Can you work these out from the model? Positions are in its coordinate system, mm. Face numbers are marked on the shaded views. A direction names the side the tool comes from. Round coordinates to 2 decimals unless told otherwise and drop trailing zeros. Loops run counter-clockwise (first coordinate to the right, second up) from the corner with the lowest first, then second, coordinate; pieces in that order, holes last. Notation, with made-up numbers: M 36.25,21.5 L 82.25,21.5 A26 ccw 82.25,56.5 Z; hole C 75,-37 d6. An arc over 180 degrees is marked long. Return JSON: item names as keys, results as strings.
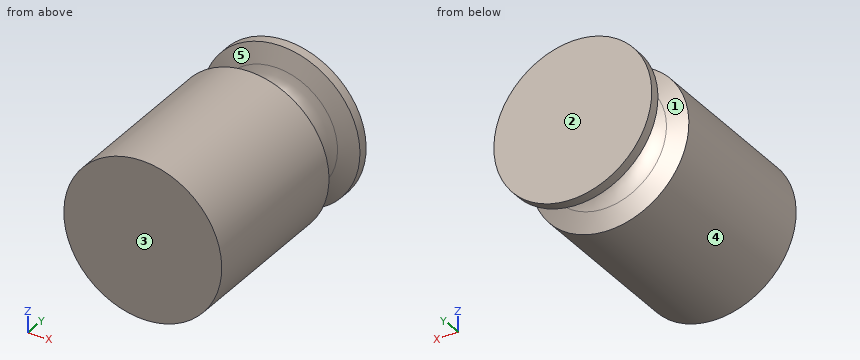
```python
from build123d import *

# Parameters (mm, degrees)
SKETCH1_R           = 25
BOSS_EXTRUDE1_DEPTH = 70


with BuildPart() as part:
    # Sketch1 → Boss-Extrude1 (new body)
    with BuildSketch(Plane(origin=(0, 0, 0), x_dir=(1, 0, 0), z_dir=(0, 1, 0))):
        with Locations(Location((0, 0, 0), (0, 0, 270))):
            Circle(SKETCH1_R)
    extrude(amount=BOSS_EXTRUDE1_DEPTH)

    # Sketch2 → Cut-Revolve3 (revolve, cut)
    with BuildSketch(Plane.XY, mode=Mode.PRIVATE) as cut_revolve3_sk:
        with BuildLine():
            Line((-25, 67), (-19.206969312, 65))
            add(Edge.make_bspline(
                [(-19.206969312, 65), (-10.627743926, 62.513316988), (-9.9009432, 56.486683012), (-19.206969312, 54)],
                knots=[0, 0, 0, 0, 1, 1, 1, 1], degree=3))
            Line((-19.206969312, 54), (-25, 52))
            Line((-25, 52), (-25, 67))
        make_face()
    revolve(cut_revolve3_sk.sketch.rotate(Axis((0, 70, 0), (0, -1, 0)), 270), axis=Axis((0, 70, 0), (0, -1, 0)), mode=Mode.SUBTRACT)


solid = part.part
```
Q1. Thinking about a two-plate mould opening in Y: for the marked faces 1, 2 and 3, which applies, pulls with the +Y half, pulls with the -Y half, needs draft (parallel to the pull), parting line crosses it, or undercut?
Results:
{"face 1": "undercut", "face 2": "pulls with the +Y half", "face 3": "pulls with the -Y half"}
Q2. On a 3-axis mill with a long thin cutter (end or side, diameter ignored), from which of +Z, -Z, +X, -X, +Y, -Y can I reach the whole of each face in a straight line? I mean the marked faces 4 and 5. Say none if no direction works.
Results:
{"face 4": "+Y, -Y", "face 5": "none"}
Q3. Suppose I cut it at A-A, the plane y = 32.5. Please give me the cut outline in (x, z).
Results:
{"outline": "C 0,0 d50"}
Q4. If I drill on line 1 along Y through (x, z) = (-18.5, 2.5); line 2 along Y through (x, z) = (-21.5, 12); line 3 along X through (y, z) = (44.5, 9), over which ranges is the centre line in solid material (lowest first)?
Results:
{"line 1": "y = 0 to 54.15, 64.84 to 70", "line 2": "y = 0 to 52.13, 66.87 to 70", "line 3": "x = -23.32 to 23.32"}
Q5. I'm going to push flat-ended pins straight in: pin 1 Ø5 at (x, y) = (-19, 48.5) entering from +Z; pin 2 Ø4 at (x, y) = (-16, 36) entering from -Z; pin 3 Ø4 at (y, z) = (8.5, -7) entering from +X; pin 4 Ø5 at (x, y) = (1.5, 15) entering from -Z. Where does each tip first touch, or does it pass through?
Results:
{"pin 1": "stops at z = 18.78", "pin 2": "stops at z = -20.71", "pin 3": "stops at x = 24.49", "pin 4": "stops at z = -25"}
